```python
from build123d import *

# Parameters (mm, degrees)
F1_DEPTH  = 6
F2_R      = 6
F2_R_2    = 3.25
F3_DEPTH  = 1.5
F4_W      = 8
F4_H      = 5
F4_W_2    = 6
F4_H_2    = 2.5
F4_W_3    = 5
F5_DEPTH  = 6.001
F6_R      = 10
F7_SIZE   = 1
F8_R      = 1.75
F9_DEPTH  = 14.5
F10_R     = 1.75
F11_DEPTH = 14.5
F12_R     = 1.7
F13_DEPTH = 6.001
F14_R     = 1.7
F15_DEPTH = 6.001
F16_W     = 6
F16_H     = 6
F16_R     = 1.7
F17_DEPTH = 2


with BuildPart() as f1:
    # F0 (on Front) → F1 (new body)
    with BuildSketch(Plane.XZ):
        with BuildLine():
            Line((-75, 0), (75, 0))
            Line((75, 0), (75, 35))
            Line((75, 35), (58.3095189485, 35))
            ThreePointArc((58.3095189485, 35), (0, 15), (-58.3095189485, 35))
            Line((-58.3095189485, 35), (-75, 35))
            Line((-75, 35), (-75, 0))
        make_face()
    extrude(amount=F1_DEPTH)

    # F2 (on face) → F3 (cut)
    with BuildSketch(Plane.XZ.offset(6)):
        with Locations((-65, 26)):
            Circle(F2_R)
        with Locations((-65, 26)):
            Circle(F2_R_2, mode=Mode.SUBTRACT)
        with Locations((65, 26)):
            Circle(F2_R)
        with Locations((65, 26)):
            Circle(F2_R_2, mode=Mode.SUBTRACT)
    extrude(amount=-F3_DEPTH, mode=Mode.SUBTRACT)

    # F4 (on face) → F5 (cut, through all)
    with BuildSketch(Plane.XZ.offset(6)):
        with Locations((-64, 2.5)):
            Rectangle(F4_W, F4_H)
        with Locations((64, 2.5)):
            Rectangle(F4_W, F4_H)
        with Locations((-64, 14.75)):
            Rectangle(F4_W_2, F4_H_2)
        with Locations((64, 14.75)):
            Rectangle(F4_W_2, F4_H_2)
        with Locations((-52.5, 2.5)):
            Rectangle(F4_W_3, F4_H)
        with Locations((52.5, 2.5)):
            Rectangle(F4_W_3, F4_H)
    extrude(amount=-F5_DEPTH, mode=Mode.SUBTRACT)

    # F6
    f6_edges = [f1.edges().sort_by_distance(p)[0] for p in [
        (-75, -3, 35),
        (75, -3, 35),
        (58.309519, -3, 35),
        (-58.309519, -3, 35),
    ]]
    fillet(f6_edges, radius=F6_R)

    # F7
    f7_edges = [f1.edges().sort_by_distance(p)[0] for p in [
        (-68, -3, 0),
        (-60, -3, 0),
        (60, -3, 0),
        (68, -3, 0),
        (-55, -3, 0),
        (-50, -3, 0),
        (50, -3, 0),
        (55, -3, 0),
    ]]
    chamfer(f7_edges, length=F7_SIZE)

    # F8 (on face) → F9 (cut)
    with BuildSketch(Plane(origin=(0, 0, 5), x_dir=(1, 0, 0), z_dir=(0, 0, -1))):
        with Locations((-64, 3)):
            Circle(F8_R)
    extrude(amount=-F9_DEPTH, mode=Mode.SUBTRACT)

    # F10 (on face) → F11 (cut)
    with BuildSketch(Plane(origin=(0, 0, 5), x_dir=(1, 0, 0), z_dir=(0, 0, -1))):
        with Locations((64, 3)):
            Circle(F10_R)
    extrude(amount=-F11_DEPTH, mode=Mode.SUBTRACT)

    # F12 (on face) → F13 (cut, through all)
    with BuildSketch(Plane.XZ.offset(6)):
        with Locations((-65, 26)):
            Circle(F12_R)
    extrude(amount=-F13_DEPTH, mode=Mode.SUBTRACT)

    # F14 (on face) → F15 (cut, through all)
    with BuildSketch(Plane.XZ.offset(6)):
        with Locations((65, 26)):
            Circle(F14_R)
    extrude(amount=-F15_DEPTH, mode=Mode.SUBTRACT)

    # F16 (on face) → F17 (cut)
    with BuildSketch(Plane(origin=(0, 0, 0), x_dir=(-1, 0, 0), z_dir=(0, 1, 0))):
        with Locations((65, 26)):
            Rectangle(F16_W, F16_H)
        with Locations((65, 26)):
            Circle(F16_R, mode=Mode.SUBTRACT)
        with Locations((-65, 26)):
            Rectangle(F16_W, F16_H)
        with Locations((-65, 26)):
            Circle(F16_R, mode=Mode.SUBTRACT)
    extrude(amount=-F17_DEPTH, mode=Mode.SUBTRACT)


solid = f1.part
```
Geometry check sheet. Reference: the model listing, model coordinates, mm. A direction names the side the tool comes from. Give positions to 0.01 mm unless a question says otherwise; leave off trailing zeros. Write each loop counter-clockwise with the first axis right and the second up, starting at its lowest first coordinate (ties: lowest second). Pieces come first, ordered by that corner, then holes.
1) Section check C-C, the plane x = 33. Record the boundary of the cut face in (y, z), and give its area (3 significant figures).
2) Section check A-A, the plane z = 30.5. Record the boundary of the cut face in (x, y).
3) Release check for a two-part mould opening along Z. For faces 5 (the flat face through (63, -3, 35)), 6 (the flat face through (61, -3, 15)), 7 (the flat face through (64, -3, 19.5)) record: pulls with the +Z half, pulls with the -Z half, needs draft (parallel to the pull), parting line crosses it, or undercut.
4) Material ranges on L1, parallel to Z at x = -65, y = -5.55; L2, parallel to X at y = -4.35, z = 3.5; L3, parallel to Y at x = 64, z = 17.05, recorded low to high.
5) Access from +Z, -Z, +X, -X, +Y, -Y to the whole of each face (thin tool, end or side, straight path). Record for faces 1 (the flat face through (-65.4, -4.4, 13.5)), 2 (the flat face through (-63.6, -2, 24.7)), 3 (the flat face through (50, -3, 3)), 4 (the flat face through (-62, -4.5, 23)).
6) Section check B-B, the plane y = -3. State how many separate pieces and enclosed holes the cut face has, and give its area (3 significant figures).
7) Gauge pin test, flat ends, axial feed: pin 1 (1.5 mm diameter, centred on x = -0.5, y = -2.5, fed in from +Z); pin 2 (1 mm diameter, centred on y = -1, z = 26, fed in from -X); pin 3 (0.6 mm diameter, centred on y = -1, z = 26, fed in from +X). Record the tip position at first contact, or that the pin passes through.
8) Section check D-D, the plane z = 21.5. Record the boundary of the cut face in (x, y), and give its area (3 significant figures).
Computed:
1. outline: (-6, 0) - (0, 0) - (0, 20.92) - (-6, 20.92) - close
1. area: 125 mm2
2. outline: (-73.35, -6) - (-68.97, -6) - (-68.97, -4.5) - (-61.03, -4.5) - (-61.03, -6) - (-52.01, -6) - (-52.01, 0) - (-73.35, 0) - close; (52.01, -6) - (61.03, -6) - (61.03, -4.5) - (68.97, -4.5) - (68.97, -6) - (73.35, -6) - (73.35, 0) - (52.01, 0) - close
3. face 5: pulls with the +Z half
3. face 6: undercut
3. face 7: pulls with the -Z half
4. L1: z = 5 to 13.5, 16 to 20, 22.75 to 24.3, 27.7 to 29.25, 32 to 35
4. L2: x = -75 to -68, -60 to -55, -50 to 50, 55 to 60, 68 to 75
4. L3: y = -6 to -4.75, -1.25 to 0
5. face 1: +Y, -Y
5. face 2: +Y
5. face 3: -Z, +Y, -Y
5. face 4: -Y
6. separate pieces: 1
6. enclosed holes: 2
6. area: 3,350 mm2
7. pin 1: stops at z = 15.01
7. pin 2: stops at x = -74.99
7. pin 3: stops at x = 74.98
8. outline: (-75, -6) - (-68.97, -6) - (-68.97, -4.5) - (-61.03, -4.5) - (-61.03, -6) - (-34.54, -6) - (-34.54, 0) - (-75, 0) - close; (34.54, -6) - (61.03, -6) - (61.03, -4.5) - (68.97, -4.5) - (68.97, -6) - (75, -6) - (75, 0) - (34.54, 0) - close
8. area: 462 mm2
